Verification items for the finished model (mm, model axes). A direction names the side the tool comes from. Coordinates: 2 decimals unless noted, no trailing zeros. Loops run counter-clockwise (first coordinate to the right, second up) from the corner with the lowest first, then second, coordinate; pieces in that order, holes last.
Q1. Sectioned sample at A-A (z = 0). Enter the section's corners in (x, y).
Q2. Sectioned sample at B-B (x = 0). Enter the section's corners in (y, z), then the cut area to 3 significant figures.
Q3. Sectioned sample at D-D (y = 5.75). Enter the section's corners in (x, z).
Q4. Go/stop test with flat-tipped pins: P1, Ø8, axis at y = 8.5, z = 2.5, coming from the -X side; P2, Ø1, axis at x = -14, y = 19, coming from the -Z side; P3, Ø1, axis at x = 6, z = -3.5, coming from the -Y side; P4, Ø6, axis at y = 10, z = -1.5, coming from the +X side. Record where each tip stops, or that it passes through.
Q5. Access from +Z, -Z, +X, -X, +Y, -Y to the whole of each face (thin tool, end or side, straight path). Record for faces 1 (the face through (-25, 1, 11)), 2 (the face through (-2.17, 9.89, 9.76)), 3 (the face through (16, 19, 10)), 4 (the face through (-16, 1, 10)).
Q6. Mould release check, pull along Y, two halves, no side actions. Record for faces 5 (the face through (16, 1, 10)), 6 (the face through (-6, 20, 3)), 7 (the face through (0, 2, 11)): +Y half, -Y half, draft (parallel to the pull), parting line (faces both ways), or undercut.
Q7. Material ranges on probe 1 along Z at (x, y) = (0, 1.2); probe 2 along X at (y, z) = (10.25, 0), recorded low to high.
Q8. Sectioned sample at C-C (x = 21.5). Enter the section's corners in (y, z).
```python
from build123d import *

# Parameters (mm, degrees)
SKETCH_1_R          = 10
SKETCH_1_R_2        = 6.5
EXTRUDE_1_DEPTH     = 20
SKETCH_1_W          = 50
SKETCH_1_H          = 2
EXTRUDE_1_2_DEPTH   = 20
SKETCH_2_W          = 2
SKETCH_2_H          = 16
CUT_EXTRUDE_2_DEPTH = 50
SKETCH_3_R          = 12
EXTRUDE_2_DEPTH     = 2
SKETCH_5_R          = 12
SKETCH_5_R_2        = 6.5
EXTRUDE_3_DEPTH     = 2
SKETCH_4_R          = 6.5
CUT_EXTRUDE_4_DEPTH = 2


with BuildPart() as part:
    # Sketch 1 → Extrude 1 (new body)
    with BuildSketch(Plane(origin=(0, 0, 0), x_dir=(1, 0, 0), z_dir=(0, 1, 0))):
        Circle(SKETCH_1_R)
        Circle(SKETCH_1_R_2, mode=Mode.SUBTRACT)
    extrude(amount=EXTRUDE_1_DEPTH)



with BuildPart() as body_2:
    # Sketch 1 → Extrude 1 2 (new body)
    with BuildSketch(Plane(origin=(0, 0, 0), x_dir=(1, 0, 0), z_dir=(0, 1, 0))):
        with Locations((0, -11)):
            Rectangle(SKETCH_1_W, SKETCH_1_H)
    extrude(amount=EXTRUDE_1_2_DEPTH)

    # Sketch 2 → Cut-Extrude 2 (cut)
    with BuildSketch(Plane.ZY.offset(25)):
        with Locations((11, 10)):
            Rectangle(SKETCH_2_W, SKETCH_2_H)
    extrude(amount=-CUT_EXTRUDE_2_DEPTH, mode=Mode.SUBTRACT)


with BuildPart() as part_1:
    add(part.part)

    add(body_2.part)  # Extrude 2 merges body 2
    # Sketch 3 → Extrude 2 (add)
    with BuildSketch(Plane(origin=(0, 0, 0), x_dir=(1, 0, 0), z_dir=(0, 1, 0))):
        Circle(SKETCH_3_R)
    extrude(amount=EXTRUDE_2_DEPTH)

    # Sketch 5 → Extrude 3 (add)
    with BuildSketch(Plane(origin=(0, 20, 0), x_dir=(1, 0, 0), z_dir=(0, 1, 0))):
        Circle(SKETCH_5_R)
        Circle(SKETCH_5_R_2, mode=Mode.SUBTRACT)
    extrude(amount=-EXTRUDE_3_DEPTH)

    # Sketch 4 → Cut-Extrude 4 (cut)
    with BuildSketch(Plane.XZ):
        Circle(SKETCH_4_R)
    extrude(amount=-CUT_EXTRUDE_4_DEPTH, mode=Mode.SUBTRACT)


solid = part_1.part
```
Geometry check:
1. outline: (-12, 0) - (-6.5, 0) - (-6.5, 20) - (-12, 20) - (-12, 18) - (-10, 18) - (-10, 2) - (-12, 2) - close; (6.5, 0) - (12, 0) - (12, 2) - (10, 2) - (10, 18) - (12, 18) - (12, 20) - (6.5, 20) - close
2. outline: (0, -12) - (2, -12) - (2, -10) - (18, -10) - (18, -12) - (20, -12) - (20, -6.5) - (0, -6.5) - close; (0, 6.5) - (20, 6.5) - (20, 12) - (18, 12) - (18, 10) - (2, 10) - (2, 12) - (0, 12) - close
2. area: 156 mm2
3. outline: circle Ø20 at (0, 0); hole circle Ø13 at (0, 0)
4. P1: stops at x = -10
4. P2: stops at z = 10
4. P3: stops at y = 0
4. P4: stops at x = 10
5. face 1: +Z, -Z, -X, +Y, -Y
5. face 2: none
5. face 3: +X, +Y, -Y
5. face 4: -X, +Y, -Y
6. face 5: draft
6. face 6: +Y half
6. face 7: undercut
7. probe 1: z = -12 to -6.5, 6.5 to 12
7. probe 2: x = -10 to -6.5, 6.5 to 10
8. outline: (0, 10) - (2, 10) - (2, 12) - (0, 12) - close; (18, 10) - (20, 10) - (20, 12) - (18, 12) - close
